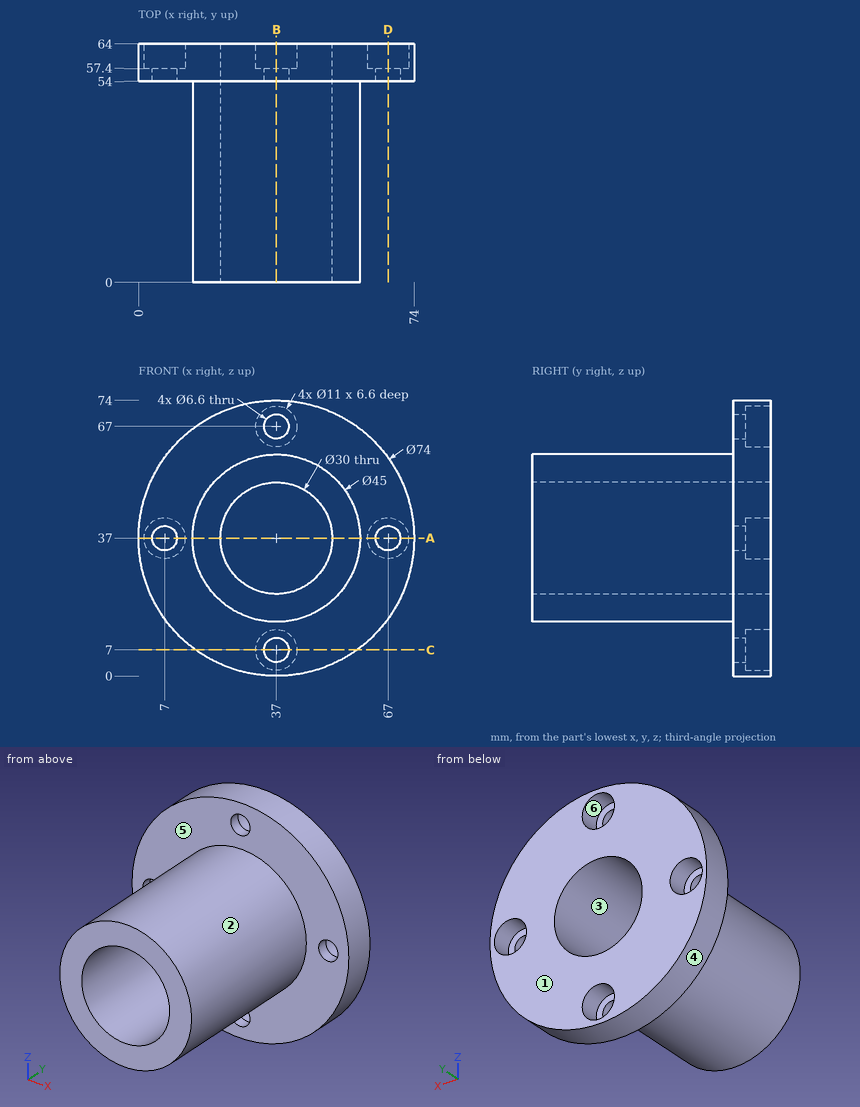
Source: three-view drawing plus pictorial views. Frame: mm from the lowest corner of the part. A direction names the side the tool comes from. Give positions to 0.01 mm unless a question says otherwise; leave off trailing zeros. Loops run counter-clockwise (first coordinate to the right, second up) from the corner with the lowest first, then second, coordinate; pieces in that order, holes last. Notation, with made-up numbers: M 43.5,-30.75 L 74.5,-30.75 A8 ccw 74.5,-23.75 Z; hole C 20,3.25 d7. An arc over 180 degrees is marked long. Use CSV: the item, a comma, the result in double quotes.
(1) Pull-direction query (X, two-part tool) for the marked faces 1, 2 and 3; classes: pulls with the +X half, pulls with the -X half, needs draft (parallel to the pull), parting line crosses it, or undercut.
Outcome:
face 1,"needs draft"
face 2,"parting line crosses it"
face 3,"undercut"
(2) Section C-C, the plane z = 7. Return loops of the section in (x, y), plus the area to 3 significant figures.
Outcome:
outline,"M 15.34,54 L 33.7,54 L 33.7,57.4 L 31.5,57.4 L 31.5,64 L 15.34,64 Z; M 40.3,54 L 58.66,54 L 58.66,64 L 42.5,64 L 42.5,57.4 L 40.3,57.4 Z"
area,"338 mm²"
(3) Section A-A, the plane z = 37. Return loops of the section in (x, y), plus the area to 3 significant figures.
Outcome:
outline,"M 0,54 L 3.7,54 L 3.7,57.4 L 1.5,57.4 L 1.5,64 L 0,64 Z; M 10.3,54 L 14.5,54 L 14.5,0 L 22,0 L 22,64 L 12.5,64 L 12.5,57.4 L 10.3,57.4 Z; M 52,0 L 59.5,0 L 59.5,54 L 63.7,54 L 63.7,57.4 L 61.5,57.4 L 61.5,64 L 52,64 Z; M 70.3,54 L 74,54 L 74,64 L 72.5,64 L 72.5,57.4 L 70.3,57.4 Z"
area,"1,060 mm²"
(4) Material intervals for L1, parallel to Z at x = 36.5, y = 58.5; L2, parallel to X at y = 55.4, z = 37; L3, parallel to Z at x = 37, y = 20, sorted ascending. Write a range as [from, to].
Outcome:
L1,"z = [0, 1.52], [12.48, 22.01], [51.99, 61.52], [72.48, 74]"
L2,"x = [0, 3.7], [10.3, 22], [52, 63.7], [70.3, 74]"
L3,"z = [14.5, 22], [52, 59.5]"
(5) Section B-B, the plane x = 37. Return loops of the section in (y, z), plus the area to 3 significant figures.
Outcome:
outline,"M 0,14.5 L 54,14.5 L 54,10.3 L 57.4,10.3 L 57.4,12.5 L 64,12.5 L 64,22 L 0,22 Z; M 0,52 L 64,52 L 64,61.5 L 57.4,61.5 L 57.4,63.7 L 54,63.7 L 54,59.5 L 0,59.5 Z; M 54,0 L 64,0 L 64,1.5 L 57.4,1.5 L 57.4,3.7 L 54,3.7 Z; M 54,70.3 L 57.4,70.3 L 57.4,72.5 L 64,72.5 L 64,74 L 54,74 Z"
area,"1,060 mm²"
(6) Pin query (flat end, axial travel): P1, Ø1, axis at x = 13.5, z = 55, coming from the -Y side; P2, Ø5.5, axis at x = 38.5, z = 8.5, coming from the +Y side; P3, Ø1.5, axis at y = 34, z = 48, coming from the +X side. Return the tip coordinate at first contact, or that it passes through.
Outcome:
P1,"stops at y = 54"
P2,"stops at y = 57.4"
P3,"stops at x = 57.03"
(7) Set-up query: the marked faces 4, 5 and 6. Return all of +Z, -Z, +X, -X, +Y, -Y with unobstructed straight access to the full face (end or side cutting, diameter ignored); none if empty.
Outcome:
face 4,"+Y, -Y"
face 5,"-Y"
face 6,"+Y"
(8) Section D-D, the plane x = 67. Return loops of the section in (y, z), plus the area to 3 significant figures.
Outcome:
outline,"M 54,15.34 L 64,15.34 L 64,31.5 L 57.4,31.5 L 57.4,33.7 L 54,33.7 Z; M 54,40.3 L 57.4,40.3 L 57.4,42.5 L 64,42.5 L 64,58.66 L 54,58.66 Z"
area,"338 mm²"
